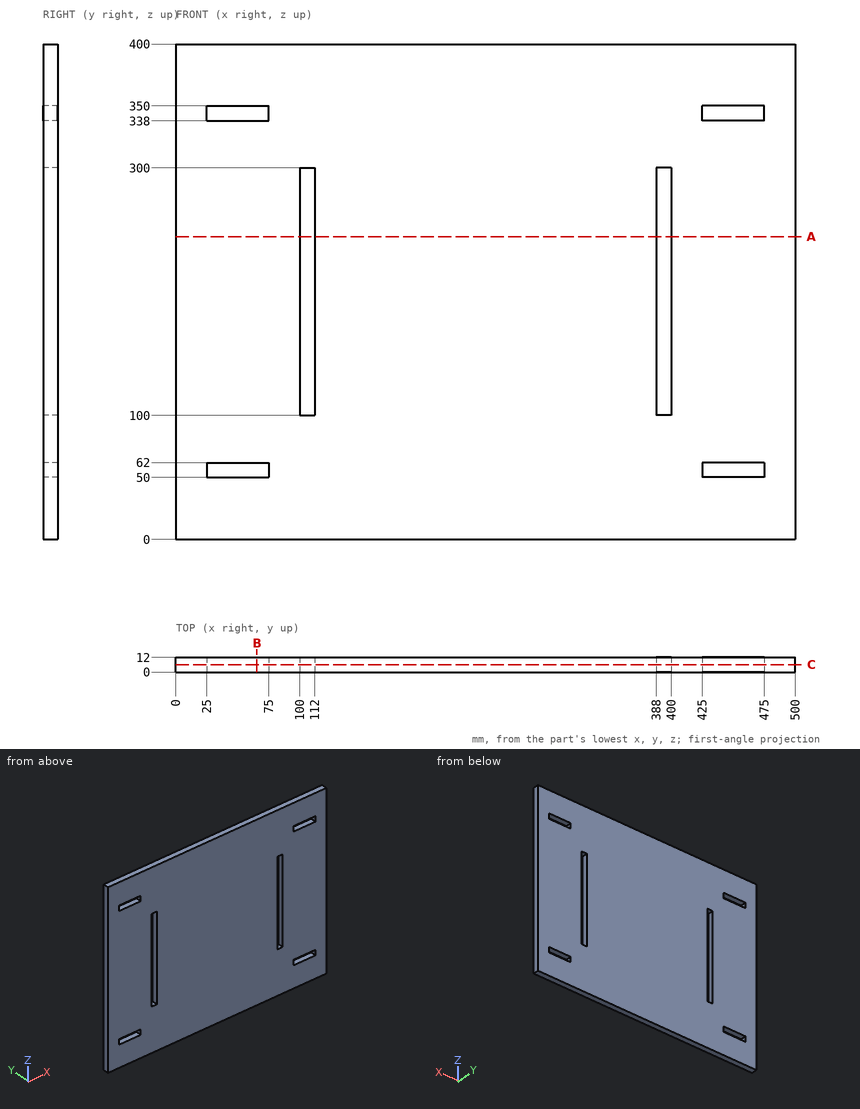
Print and shaded views of the part. All mm, measured from the part's lowest x, y and z. Give positions to 0.01 mm unless a question says otherwise; leave off trailing zeros. Write each loop counter-clockwise with the first axis right and the second up, starting at its lowest first coordinate (ties: lowest second). Pieces come first, ordered by that corner, then holes. Notation, with made-up numbers: (40, 83.25) - (54, 83.25) arc R16 cw to (54, 101.25) - close; hole circle Ø4 at (31, 14.5). An arc over 180 degrees is marked (long way). One line per question, with ' | ' between items. Start each with the question number.
(1) Slice it at A-A on z = 244.5. Write the cut outline in (x, y), plus the area to 3 significant figures.
(2) Slice it at B-B on x = 65.5. Write the cut outline in (y, z).
(3) Wall check: line 1 along X through (y, z) = (5.25, 136); line 2 along Z through (x, y) = (474.5, 8.5); line 3 along X through (y, z) = (5, 61). Give the ranges that are in metal, low to high. Write a range as from..to.
(4) Slice it at C-C on y = 6. Write the cut outline in (x, z), plus the area to 3 significant figures.
Results below:
1) outline: (0, 0) - (100, 0) - (100, 12) - (0, 12) - close; (112, 0) - (388, 0) - (388, 12) - (112, 12) - close; (400, 0) - (500, 0) - (500, 12) - (400, 12) - close | area: 5,710 mm^2
2) outline: (0, 0) - (12, 0) - (12, 50) - (0, 50) - close; (0, 62) - (12, 62) - (12, 338) - (0, 338) - close; (0, 350) - (12, 350) - (12, 400) - (0, 400) - close
3) line 1: 0..100, 112..388, 400..500 | line 2: 0..50, 62..338, 350..400 | line 3: 0..25, 75..425, 475..500
4) outline: (0, 0) - (500, 0) - (500, 400) - (0, 400) - close; hole (25, 50) - (75, 50) - (75, 62) - (25, 62) - close; hole (25, 338) - (75, 338) - (75, 350) - (25, 350) - close; hole (100, 100) - (112, 100) - (112, 300) - (100, 300) - close; hole (388, 100) - (400, 100) - (400, 300) - (388, 300) - close; hole (425, 50) - (475, 50) - (475, 62) - (425, 62) - close; hole (425, 338) - (475, 338) - (475, 350) - (425, 350) - close | area: 193,000 mm^2
